Input: part model. Units: mm. Frame: model coordinates. A direction names the side the tool comes from. Round coordinates to 2 decimals unless told otherwise and drop trailing zeros. Loops run counter-clockwise (first coordinate to the right, second up) from the corner with the lowest first, then second, coordinate; pieces in that order, holes last. Notation, with made-up numbers: (-17.5, 59) -> (4.5, 59) arc R33 ccw to (4.5, 91) -> close; hole circle Ø4 at (55.25, -8). An arc over 180 degrees is marked (long way). Answer as a JSON object with one key per item and string values. Group by question number.
Item 1: Draft query along Y for faces 4 (the flat face through (39.9, 14, 3)), 5 (the flat face through (145, 5.6, 3)), 6 (the flat face through (125, 11, 3)). Return one class per face: released by +Y, released by -Y, zero draft, split by the parting line, or undercut.
Item 2: Set-up query: faces 1 (the flat face through (65, 11, 3)), 2 (the flat face through (25, -71.6, 3)), 3 (the flat face through (145, -77, 3)). Return all of +Z, -Z, +X, -X, +Y, -Y with unobstructed straight access to the full face (end or side cutting, diameter ignored); none if empty.
Item 3: Pin query (flat end, axial travel): pin 1 (3 mm diameter, centred on x = 174.5, z = 3, fed in from +Y); pin 2 (3 mm diameter, centred on y = 13, z = 3.5, fed in from +X). Return the tip coordinate at first contact, or that it passes through.
Item 4: Section query B-B on z = 1.15. Count the separate pieces of the cut face and the enclosed holes in it, and give its area (3 significant figures).
Item 5: Section query C-C on x = 67. Return loops of the section in (y, z), and give its area (3 significant figures).
Item 6: Section query A-A on x = 24.5. Return loops of the section in (y, z).
Item 7: Material intervals for line 1 (Y direction, x = 86, z = 3.75); line 2 (Y direction, x = 40, z = 0.4), sorted ascending. Write a range as [from, to].
Autodesk Inventor part; units mm, degrees
ref_plane "YZ Plane" through (0, 0, 0) normal (1, 0, 0) x (0, 1, 0)
ref_plane "XZ Plane" through (0, 0, 0) normal (0, 1, 0) x (-1, 0, 0)
ref_plane "XY Plane" through (0, 0, 0) normal (0, 0, 1) x (1, 0, 0)
sketch "Sketch1" plane through (0, 0, 0) normal (0, 0, 1) x (1, 0, 0)
  line L0 (184.3024, 11) -> (184.3024, 17)
  line L1 (-10, 11) -> (-10, 17)
  line L2 (184.3024, 17) -> (0, 17)
  line L3 (0, 17) -> (0, -83)
  line L4 (0, -83) -> (184.3024, -83)
  line L5 (184.3024, -83) -> (184.3024, 17)
  line L6 (-10, 17) -> (0, 17)
  line L7 (0, 17) -> (0, -83)
  line L8 (0, -83) -> (-10, -83)
  line L9 (-10, -83) -> (-10, 17)
  point P0 (0, 0)
  point P1 (-10, 6)
  point P2 (-10, 0)
  dimension "d0" = 100
extrude "Extrusion1" add sketch "Sketch1" along normal blind 6
sketch "Sketch4" plane through (0, 0, 6) normal (0, 0, 1) x (1, 0, 0)
  line L0 (160, 11) -> (184.3024, 11)
  line L1 (160, 17) -> (160, 11)
  line L2 (184.3024, 17) -> (-10, 17)
  line L3 (184.3024, -83) -> (184.3024, 17)
  line L4 (0, 11) -> (-10, 11)
  line L5 (0, 17) -> (0, 0)
  line L6 (-10, 17) -> (-10, -83)
  point P0 (-10, 11)
extrude "Extrusion4" cut sketch "Sketch4" against normal blind 6 contours L1 L2 L3 L0
sketch "Sketch5" plane through (0, 0, 6) normal (0, 0, 1) x (1, 0, 0)
  line L0 (140, 11) -> (150, 11)
  line L1 (150, 11) -> (150, 17)
  line L2 (140, 17) -> (140, 11)
  line L3 (184.3024, 17) -> (-10, 17)
  line L4 (150, 11) -> (150.1, 11)
  line L5 (150.1, 11) -> (150.1, 17)
  line L6 (150.1, 17) -> (150, 17)
  line L7 (150, 17) -> (150, 11)
  line L8 (140, 11) -> (139.9, 11)
  line L9 (139.9, 11) -> (139.9, 17)
  line L10 (139.9, 17) -> (140, 17)
  line L11 (140, 17) -> (140, 11)
  point P0 (0, 0)
  point P1 (160, 17)
  point P2 (0, 6)
  point P3 (150.1, 17)
  point P4 (139.9, 17)
  point P5 (-10, 17)
  point P6 (184.3024, 17)
  dimension "d21" = 0.1
  dimension "d22" = 6
  dimension "d23" = 0.1
  dimension "d24" = 6
extrude "Extrusion5" cut sketch "Sketch5" against normal blind 6
pattern_linear "Rectangular Pattern3" count 8 spacing 20 along (-1, 0, 0) of "Extrusion5"
ref_plane "Work Plane1" through (-10, -33, 0) normal (0, -1, 0) x (1, 0, 0)
mirror "Mirror1" about plane through (-10, -33, 0) normal (0, -1, 0) of "Extrusion5"
pattern_linear "Rectangular Pattern4" count 2 spacing 20 along (1, 0, 0) count 8 spacing 20 along (-1, 0, 0) of "Extrusion5", "Mirror1"
sketch "Sketch6" plane through (0, 0, 6) normal (0, 0, 1) x (1, 0, 0)
  line L0 (167.75, 6.6) -> (162.25, 6.6)
  line L1 (162.25, 6.6) -> (162.25, 9)
  line L2 (162.25, 9) -> (167.75, 9)
  line L3 (167.75, 9) -> (167.75, 6.6)
  line L4 (159.9, 11) -> (159.9, 17)
  line L5 (184.3024, 11) -> (160, 11)
  line L6 (147.75, 5.6) -> (142.25, 5.6)
  line L7 (142.25, 5.6) -> (142.25, 8)
  line L8 (142.25, 8) -> (147.75, 8)
  line L9 (147.75, 8) -> (147.75, 5.6)
  line L10 (150.1, 11) -> (139.9, 11)
  line L11 (139.9, 11) -> (139.9, 17)
  point P0 (0, 0)
  dimension "d36" = 5.5
  dimension "d37" = 2.4
  dimension "d38" = 2.35
  dimension "d39" = 2
  dimension "d48" = 5.5
  dimension "d49" = 2.4
  dimension "d50" = 3
  dimension "d51" = 2.35
extrude "Extrusion6" cut sketch "Sketch6" against normal blind 6 contours L6 L7 L8 L9
pattern_linear "Rectangular Pattern5" count 3 spacing 60 along (-1, 0, 0) of "Extrusion6"
mirror "Mirror2" about plane through (-10, -33, 0) normal (0, -1, 0) of "Extrusion6", "Rectangular Pattern5"
properties part number "00_Baseplate_Simmo_side5_v2"
Solved:
{
 "1": {"face 4": "zero draft", "face 5": "undercut", "face 6": "released by +Y"},
 "2": {"face 1": "+Z, -Z, +Y", "face 2": "+Z, -Z", "face 3": "+Z, -Z, -Y"},
 "3": {"pin 1": "y = 11", "pin 2": "x = 159.9"},
 "4": {"separate pieces": "1", "enclosed holes": "6", "area": "18,200 mm²"},
 "5": {"outline": "(-77, 0) -> (11, 0) -> (11, 6) -> (-77, 6) -> close", "area": "528 mm²"},
 "6": {"outline": "(-77, 0) -> (-74, 0) -> (-74, 6) -> (-77, 6) -> close; (-71.6, 0) -> (5.6, 0) -> (5.6, 6) -> (-71.6, 6) -> close; (8, 0) -> (11, 0) -> (11, 6) -> (8, 6) -> close"},
 "7": {"line 1": "[-77, -74], [-71.6, 5.6], [8, 11]", "line 2": "[-77, 11]"}
}
